Read the model definition and answer for the solid it produces. Units are mm, in the model's axes. Coordinates: 2 decimals unless noted, no trailing zeros. Write each loop counter-clockwise with the first axis right and the second up, starting at its lowest first coordinate (ties: lowest second). Pieces come first, ordered by that corner, then holes. Notation, with made-up numbers: (42, 71.5) - (92, 71.5) arc R13 ccw to (92, 86.5) - close; hole circle Ø7 at (-28.75, -16.5). An arc over 180 degrees is marked (long way). Return JSON: item names as keys, results as strings.
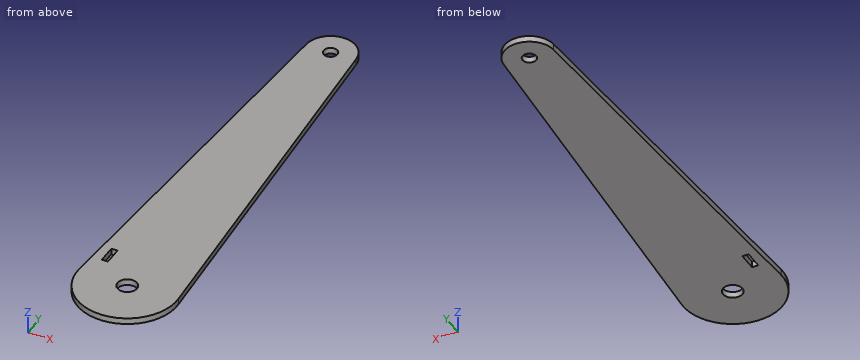
```python
from build123d import *

# Parameters (mm, degrees)
SKETCH1_R           = 4.953
SKETCH1_R_2         = 3.5
SKETCH1_W           = 3.175
SKETCH1_H           = 9.525
BOSS_EXTRUDE1_DEPTH = 3.175


with BuildPart() as part:
    # Sketch1 → Boss-Extrude1 (new body)
    with BuildSketch(Plane.XY):
        with BuildLine():
            Line((-25.350535869, 1.58440246), (-12.7, 203.993746978))
            ThreePointArc((-12.7, 203.993746978), (0, 215.924780323), (12.7, 203.993746978))
            Line((12.7, 203.993746978), (25.350535869, 1.58440246))
            ThreePointArc((25.350535869, 1.58440246), (0, -25.4), (-25.350535869, 1.58440246))
        make_face()
        Circle(SKETCH1_R, mode=Mode.SUBTRACT)
        with Locations((0, 203.2)):
            Circle(SKETCH1_R_2, mode=Mode.SUBTRACT)
        with Locations((-17.9197, 17.4625)):
            Rectangle(SKETCH1_W, SKETCH1_H, mode=Mode.SUBTRACT)
    extrude(amount=BOSS_EXTRUDE1_DEPTH)


solid = part.part
```
(1) A cutting plane is placed at A-A (x = 0). Determine the outline of the cut face in (y, z) (3 decimals).
Answer:
{"outline": "(-25.4, 0) - (-4.953, 0) - (-4.953, 3.175) - (-25.4, 3.175) - close; (4.953, 0) - (199.7, 0) - (199.7, 3.175) - (4.953, 3.175) - close; (206.7, 0) - (215.925, 0) - (215.925, 3.175) - (206.7, 3.175) - close"}
(2) A cutting plane is placed at C-C (y = 95). Determine the outline of the cut face in (x, z) (3 decimals).
Answer:
{"outline": "(-19.512, 0) - (19.512, 0) - (19.512, 3.175) - (-19.512, 3.175) - close"}
(3) Straight lines are drawn through the part: line 1 (Y direction, x = 0, z = 1.55); line 2 (X direction, y = 203.2, z = 1.5); line 3 (Y direction, x = 1.5, z = 0.8). For each, find the intervals that lie inside material, in ascending order. Write a range as from..to.
Answer:
{"line 1": "-25.4..-4.95, 4.95..199.7, 206.7..215.92", "line 2": "-12.75..-3.5, 3.5..12.75", "line 3": "-25.36..-4.72, 4.72..200.04, 206.36..215.84"}
(4) Flat-ended cylindrical pins translate along their axes: P1, Ø1.6, axis at y = 17.5, z = 1, coming from the -X side; P2, Ø1, axis at x = -17.5, z = 2, coming from the -Y side; P3, Ø6, axis at x = 0, y = 0, coming from the +Z side. Find the tip coordinate at first contact, or state that the pin passes through.
Answer:
{"P1": "x = -24.41", "P2": "y = -18.87", "P3": "through"}
(5) A cutting plane is placed at D-D (x = 16.5). Determine the outline of the cut face in (y, z) (3 decimals), and give its area (3 significant figures).
Answer:
{"outline": "(-19.311, 0) - (143.194, 0) - (143.194, 3.175) - (-19.311, 3.175) - close", "area": "516 mm²"}
(6) A cutting plane is placed at B-B (z = 0.5). Determine the outline of the cut face in (x, y) (3 decimals), and give its area (3 significant figures).
Answer:
{"outline": "(-25.351, 1.584) arc R25.4 ccw (long way) to (25.351, 1.584) - (12.7, 203.994) arc R12.725 ccw to (-12.7, 203.994) - close; hole (-19.507, 12.7) - (-16.332, 12.7) - (-16.332, 22.225) - (-19.507, 22.225) - close; hole circle Ø9.906 at (0, 0); hole circle Ø7 at (0, 203.2)", "area": "8,880 mm²"}
